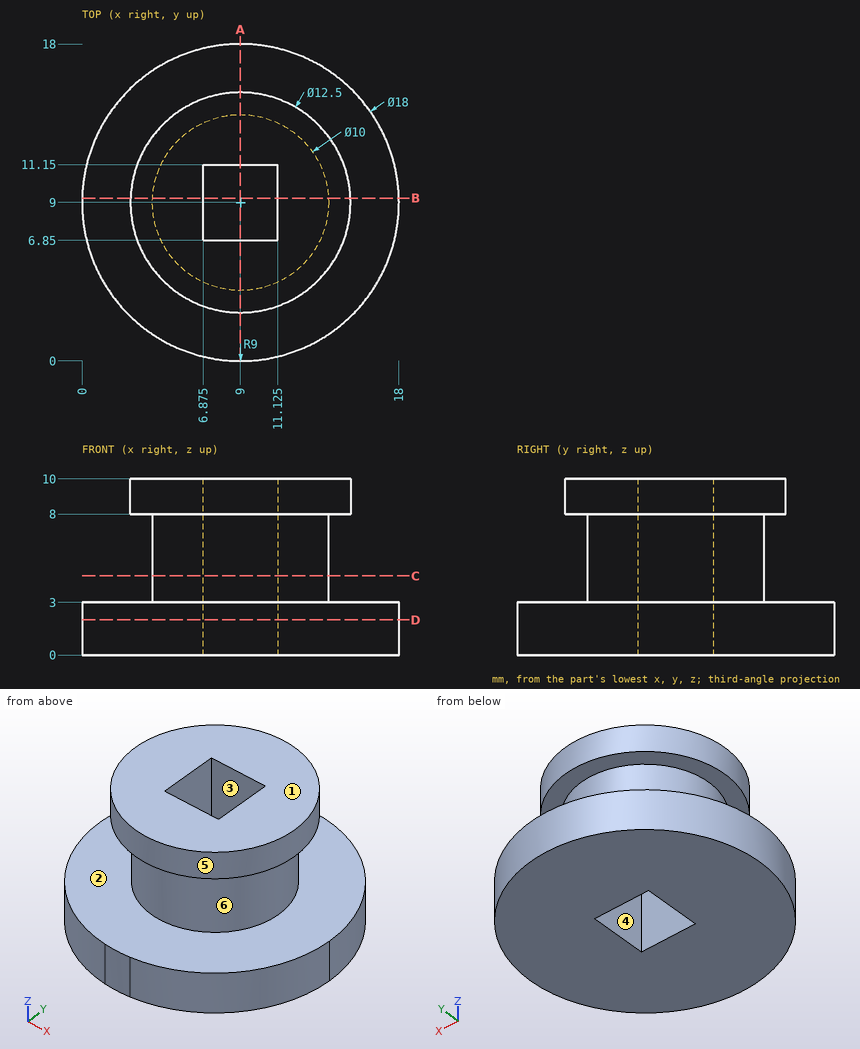
Could you check a few things on this drawing? It's one solid part, dimensions in mm from its lowest x, y, z. A direction names the side the tool comes from. Round coordinates to 2 decimals unless told otherwise and drop trailing zeros. Order: outer loops, then holes, each group sorted by start corner. A loop starts at its lowest first (then second) coordinate and runs counter-clockwise, first axis right, second up. Notation, with made-up numbers: M 23.5,45.5 L 40.5,45.5 A20 cw 40.5,83.5 Z; hole C -36,59.25 d6. An arc over 180 degrees is marked long. One line per item, written item: value.
(1) Imagine slicing it at A-A (x = 9). Write out the boundary of the cut face in (y, z), and give its area (3 significant figures).
Ans:
outline: M 0,0 L 6.85,0 L 6.85,10 L 2.75,10 L 2.75,8 L 4,8 L 4,3 L 0,3 Z; M 11.15,0 L 18,0 L 18,3 L 14,3 L 14,8 L 15.25,8 L 15.25,10 L 11.15,10 Z
area: 86.0 mm^2
(2) Which directions (+Z, -Z, +X, -X, +Y, -Y) give clear straight access to the entire face, cutting with the end or side of a thin tool? Please do the marked faces 4, 5 and 6.
Ans:
face 4: +Z, -Z
face 5: +Z
face 6: none
(3) Imagine slicing it at D-D (z = 2). Write out the boundary of the cut face in (x, y) (3 decimals).
Ans:
outline: M 8,0.056 A9 ccw 10,0.056 A9 ccw long Z; hole M 6.875,6.85 L 11.125,6.85 L 11.125,11.15 L 6.875,11.15 Z
(4) Imagine slicing it at B-B (y = 9.25). Write out the boundary of the cut face in (x, z) (1 decimal), and give its area (3 significant figures).
Ans:
outline: M 0,0 L 6.9,0 L 6.9,10 L 2.8,10 L 2.8,8 L 4,8 L 4,3 L 0,3 Z; M 11.1,0 L 18,0 L 18,3 L 14,3 L 14,8 L 15.2,8 L 15.2,10 L 11.1,10 Z
area: 86.4 mm^2
(5) I need wall thicknesses on line 1 along Z through (x, y) = (5, 13); line 2 along X through (y, z) = (9, 4.75) (3 decimals); line 3 along Y through (x, z) = (10.5, 7). Which ranges of each line are inside material? Lowest first, please. Write a range as from..to.
Ans:
line 1: z = 0..3, 8..10
line 2: x = 4..6.875, 11.125..14
line 3: y = 4.23..6.85, 11.15..13.77
(6) Imagine slicing it at C-C (z = 4.5). Write out the boundary of the cut face in (x, y) (3 decimals).
Ans:
outline: C 9,9 d10; hole M 6.875,6.85 L 11.125,6.85 L 11.125,11.15 L 6.875,11.15 Z
(7) If we mould it in two halves opening along Z, with no side actions, what happens to the marked faces 1, 2 and 3? For each: released by +Z, released by -Z, zero draft, split by the parting line, or undercut.
Ans:
face 1: released by +Z
face 2: undercut
face 3: zero draft
(8) I'm going to push flat-ended pins straight in: P1, Ø2, axis at y = 3.5, z = 3, coming from the +X side; P2, Ø2, axis at y = 12, z = 8.5, coming from the +X side. Where does each tip first touch, or does it pass through?
Ans:
P1: stops at x = 16.79
P2: stops at x = 14.92
